from build123d import *

# Parameters (mm, degrees)
SKETCH1_R           = 1.4224
BOSS_EXTRUDE1_DEPTH = 2.9718


with BuildPart() as part:
    # Sketch1 → Boss-Extrude1 (new body)
    with BuildSketch(Plane.XY):
        Polygon((25.4, 25.4), (2.9718, 25.4), (2.9718, 16.256), (0, 16.256), (0, 9.144), (2.9718, 9.144), (2.9718, 0), (9.2075, 0), (9.2075, 2.9718), (11.2395, 2.9718), (11.2395, 5.08), (9.2075, 5.08), (9.2075, 7.62), (11.2395, 7.62), (11.2395, 10.16), (14.1605, 10.16), (14.1605, 7.62), (16.1925, 7.62), (16.1925, 5.08), (14.1605, 5.08), (14.1605, 2.9718), (16.1925, 2.9718), (16.1925, 0), (25.4, 0), align=None)
        with Locations((1.4859, 12.7)):
            Circle(SKETCH1_R, mode=Mode.SUBTRACT)
    extrude(amount=BOSS_EXTRUDE1_DEPTH)


solid = part.part
Could you check a few things on this model? Use its own coordinates, in mm. A direction names the side the tool comes from. Give positions to 0.01 mm unless a question says otherwise; leave off trailing zeros. Write each loop counter-clockwise with the first axis right and the second up, starting at its lowest first coordinate (ties: lowest second). Pieces come first, ordered by that corner, then holes. Notation, with made-up numbers: (36, 71.5) - (44, 71.5) arc R11 ccw to (44, 87.5) - close; hole circle Ø8 at (81.25, 88.25). An arc over 180 degrees is marked (long way). Use CSV: the item, a comma, the result in double quotes. Start each with the question number.
Item 1: I want a section at D-D, the plane x = 12.75. Please give me the cut outline in (y, z).
Item 2: If we mould it in two halves opening along Y, with no side actions, what happens to faces 1 (the face through (14, 25.4, 1)), 2 (the face through (16.192, 6, 1)), 3 (the face through (13, 13, 0)), 4 (the face through (15, 2.972, 1))? For each: pulls with the +Y half, pulls with the -Y half, needs draft (parallel to the pull), parting line crosses it, or undercut.
Item 3: I'm going to push flat-ended pins straight in: pin 1 (0.9 mm diameter, centred on x = 13, z = 1.5, fed in from -Y); pin 2 (0.6 mm diameter, centred on y = 4.5, z = 1.5, fed in from -X); pin 3 (1 mm diameter, centred on x = 15, z = 2, fed in from -Y). Where does each tip first touch, or does it pass through?
Item 4: For faces 5 (the face through (1, 9.144, 1)), 6 (the face through (13, 10.16, 1)), 7 (the face through (10, 5.08, 1)), 8 (the face through (2.972, 21, 1)), which set-ups out of +Z, -Z, +X, -X, +Y, -Y let a thin tool reach every point of the face, with its end or its side?
Item 5: I want a section at C-C, the plane x = 10. Please give me the cut outline in (y, z), then the cut area to 3 significant figures.
Item 6: I want a section at A-A, the plane y = 12.7. Please give me the cut outline in (x, z), then the cut area to 3 significant figures.
Item 7: I want a section at B-B, the plane z = 0.8. Please give me the cut outline in (x, y), then the cut area to 3 significant figures.
Item 8: If I drill on line 1 along X through (y, z) = (10, 2.8); line 2 along X through (y, z) = (5.75, 1.15); line 3 along Y through (x, z) = (10, 2.7), over which ranges is the centre line in solid material (lowest first)?
Findings:
1,outline,"(10.16, 0) - (25.4, 0) - (25.4, 2.97) - (10.16, 2.97) - close"
2,face 1,"pulls with the +Y half"
2,face 2,"undercut"
2,face 3,"needs draft"
2,face 4,"pulls with the -Y half"
3,pin 1,"stops at y = 10.16"
3,pin 2,"stops at x = 2.97"
3,pin 3,"stops at y = 2.97"
4,face 5,"+Z, -Z, -X, -Y"
4,face 6,"+Z, -Z, -Y"
4,face 7,"+Z, -Z"
4,face 8,"+Z, -Z, -X, +Y"
5,outline,"(2.97, 0) - (5.08, 0) - (5.08, 2.97) - (2.97, 2.97) - close; (7.62, 0) - (25.4, 0) - (25.4, 2.97) - (7.62, 2.97) - close"
5,area,"59.1 mm2"
6,outline,"(0, 0) - (0.06, 0) - (0.06, 2.97) - (0, 2.97) - close; (2.91, 0) - (25.4, 0) - (25.4, 2.97) - (2.91, 2.97) - close"
6,area,"67.0 mm2"
7,outline,"(0, 9.14) - (2.97, 9.14) - (2.97, 0) - (9.21, 0) - (9.21, 2.97) - (11.24, 2.97) - (11.24, 5.08) - (9.21, 5.08) - (9.21, 7.62) - (11.24, 7.62) - (11.24, 10.16) - (14.16, 10.16) - (14.16, 7.62) - (16.19, 7.62) - (16.19, 5.08) - (14.16, 5.08) - (14.16, 2.97) - (16.19, 2.97) - (16.19, 0) - (25.4, 0) - (25.4, 25.4) - (2.97, 25.4) - (2.97, 16.26) - (0, 16.26) - close; hole circle Ø2.84 at (1.49, 12.7)"
7,area,"532 mm2"
8,line 1,"x = 0 to 11.24, 14.16 to 25.4"
8,line 2,"x = 2.97 to 9.21, 16.19 to 25.4"
8,line 3,"y = 2.97 to 5.08, 7.62 to 25.4"
